```python
from build123d import *

# Parameters (mm, degrees)
SKETCH_1_W          = 250
SKETCH_1_H          = 156
SKETCH_1_W_2        = 226
SKETCH_1_H_2        = 128
EXTRUDE_1_DEPTH     = 8
SKETCH_2_W          = 235.5
SKETCH_2_H          = 139.5
CUT_EXTRUDE_3_DEPTH = 6
CUT_EXTRUDE_4_DEPTH = 10
CUT_EXTRUDE_5_DEPTH = 10
SKETCH_6_W          = 250
SKETCH_6_H          = 156
CUT_EXTRUDE_6_DEPTH = 1


with BuildPart() as part:
    # 草图1 → 凸台-拉伸1 (new body)
    with BuildSketch(Plane(origin=(0, 0, 0), x_dir=(1, 0, 0), z_dir=(0, 1, 0))):
        with Locations((25.659327926, -14.898030127)):
            Rectangle(SKETCH_1_W, SKETCH_1_H)
        with Locations((25.659327926, -14.898030127)):
            Rectangle(SKETCH_1_W_2, SKETCH_1_H_2, mode=Mode.SUBTRACT)
    extrude(amount=EXTRUDE_1_DEPTH)

    # 草图2 → 切除-拉伸3 (cut)
    with BuildSketch(Plane.XZ):
        with Locations((24.659327926, 12.898030127)):
            Rectangle(SKETCH_2_W, SKETCH_2_H)
    extrude(amount=-CUT_EXTRUDE_3_DEPTH, mode=Mode.SUBTRACT)

    # 草图3 → 切除-拉伸4 (cut)
    with BuildSketch(Plane(origin=(0, 8, 0), x_dir=(1, 0, 0), z_dir=(0, 1, 0))):
        with BuildLine():
            Line((-89.340672074, 63.101969873), (-99.340672074, 63.101969873))
            Line((-99.340672074, 63.101969873), (-99.340672074, 53.101969873))
            ThreePointArc((-99.340672074, 53.101969873), (-96.411739886, 60.173037684), (-89.340672074, 63.101969873))
        make_face()
    extrude(amount=-CUT_EXTRUDE_4_DEPTH, mode=Mode.SUBTRACT)

    # 草图4 → 切除-拉伸5 (cut)
    with BuildSketch(Plane(origin=(0, 8, 0), x_dir=(1, 0, 0), z_dir=(0, 1, 0))):
        with BuildLine():
            Line((-99.340672074, -82.898030127), (-99.340672074, -92.898030127))
            Line((-99.340672074, -92.898030127), (-89.340672074, -92.898030127))
            ThreePointArc((-89.340672074, -92.898030127), (-96.411739886, -89.969097939), (-99.340672074, -82.898030127))
        make_face()
        with BuildLine():
            Line((150.659327926, -82.898030127), (150.659327926, -92.898030127))
            Line((150.659327926, -92.898030127), (140.659327926, -92.898030127))
            ThreePointArc((140.659327926, -92.898030127), (147.730395738, -89.969097939), (150.659327926, -82.898030127))
        make_face()
        with BuildLine():
            Line((140.659327926, 63.101969873), (150.659327926, 63.101969873))
            Line((150.659327926, 63.101969873), (150.659327926, 53.101969873))
            ThreePointArc((150.659327926, 53.101969873), (147.730395738, 60.173037684), (140.659327926, 63.101969873))
        make_face()
    extrude(amount=-CUT_EXTRUDE_5_DEPTH, mode=Mode.SUBTRACT)

    # 草图6 → 切除-拉伸6 (cut)
    with BuildSketch(Plane(origin=(0, 8, 0), x_dir=(1, 0, 0), z_dir=(0, 1, 0))):
        with Locations((25.659327926, -14.898030127)):
            Rectangle(SKETCH_6_W, SKETCH_6_H)
    extrude(amount=-CUT_EXTRUDE_6_DEPTH, mode=Mode.SUBTRACT)


solid = part.part
```
Check sheet for the modelled part. Datum: model origin and axes. Units: mm. A direction names the side the tool comes from. Round coordinates to 2 decimals unless told otherwise and drop trailing zeros. Loops run counter-clockwise (first coordinate to the right, second up) from the corner with the lowest first, then second, coordinate; pieces in that order, holes last. Notation, with made-up numbers: (-4, -14.5) - (26, -14.5) arc R22 cw to (26, -0.5) - close; hole circle Ø2 at (7, 30). An arc over 180 degrees is marked (long way). Write item = value, one per line. Start each with the question number.
Q1. Thickness scan on L1, parallel to Z at x = -24, y = 5.25; L2, parallel to X at y = 2, z = -39; L3, parallel to Z at x = 18, y = 6.5. Record the ranges inside material, lowest first.
Q2. Section check A-A (z = -39). Record the boundary of the cut face in (x, y), plus the area to 3 significant figures.
Q3. Access from +Z, -Z, +X, -X, +Y, -Y to the whole of each face (thin tool, end or side, straight path). Record for faces 1 (the face through (147.7, 3.5, 90)), 2 (the face through (-93.091, 3, 12)).
Q4. Section check C-C (x = 135). Record the boundary of the cut face in (y, z), plus the area to 3 significant figures.
Q5. Release check for a two-part mould opening along Z. For faces 3 (the face through (23, 3, 82.648)), 4 (the face through (16, 7, 84)), 5 (the face through (147.8, 3.5, -60.1)) record: pulls with the +Z half, pulls with the -Z half, needs draft (parallel to the pull), parting line crosses it, or undercut.
Q6. Section check B-B (y = 3). Record the boundary of the cut face in (x, z), plus the area to 3 significant figures.
Derived:
q1.L1 = -63.1 to -56.85, 82.65 to 92.9
q1.L2 = -99.34 to -93.09, 142.41 to 150.66
q1.L3 = -63.1 to -49.1, 78.9 to 92.9
q2.outline = (-99.34, 0) - (-93.09, 0) - (-93.09, 6) - (-87.34, 6) - (-87.34, 7) - (-99.34, 7) - close; (138.66, 6) - (142.41, 6) - (142.41, 0) - (150.66, 0) - (150.66, 7) - (138.66, 7) - close
q2.area = 111 mm^2
q3.face_1 = +Z, +X, +Y, -Y
q3.face_2 = -Y
q4.outline = (0, -63.1) - (7, -63.1) - (7, -49.1) - (6, -49.1) - (6, -56.85) - (0, -56.85) - close; (0, 82.65) - (6, 82.65) - (6, 78.9) - (7, 78.9) - (7, 92.9) - (0, 92.9) - close
q4.area = 127 mm^2
q5.face_3 = undercut
q5.face_4 = needs draft
q5.face_5 = pulls with the -Z half
q6.outline = (-99.34, -53.1) arc R10 ccw to (-89.34, -63.1) - (140.66, -63.1) arc R10 ccw to (150.66, -53.1) - (150.66, 82.9) arc R10 ccw to (140.66, 92.9) - (-89.34, 92.9) arc R10 ccw to (-99.34, 82.9) - close; hole (-93.09, -56.85) - (142.41, -56.85) - (142.41, 82.65) - (-93.09, 82.65) - close
q6.area = 6,060 mm^2
